Can you work these out from the model? Positions are in its coordinate system, mm. A direction names the side the tool comes from. Give positions to 0.01 mm unless a question says otherwise; leave off trailing zeros. Loops run counter-clockwise (first coordinate to the right, second up) from the corner with the lowest first, then second, coordinate; pieces in that order, holes last. Notation, with made-up numbers: (6, 63.25) - (16, 63.25) arc R24 cw to (16, 88.25) - close; hole circle Ø7 at (75.25, 50). An arc over 180 degrees is marked (long way). Answer as a JSON object with one key per item and string values.
```python
from build123d import *

# Parameters (mm, degrees)
F0_R     = 10.9982
F1_DEPTH = 7.0104
F2_R     = 1.27
F3_R     = 1.27


with BuildPart() as f1:
    # F0 (on Front) → F1 (new body)
    with BuildSketch(Plane.XZ):
        Polygon((-12.7, 9.9571658781), (-12.7, 5.2605122421), (-5.2605122421, 12.7), (-9.9571658781, 12.7), (-11.4818856978, 16.9197350247), (-28.3834853749, 28.3834853749), (-16.9197350247, 11.4818856978), align=None)
        Polygon((-16.0210356348, -1.9394766073), (-12.7, -5.2605122421), (-12.7, 5.2605122421), (-16.0210356348, 1.9394766073), (-20.0829786096, 3.8451401341), (-40.1403099645, 0), (-20.0829786096, -3.8451401341), align=None)
        Polygon((-9.9571658781, -12.7), (-5.2605122421, -12.7), (-12.7, -5.2605122421), (-12.7, -9.9571658781), (-16.9197350247, -11.4818856978), (-28.3834853749, -28.3834853749), (-11.4818856978, -16.9197350247), align=None)
        Polygon((1.9394766073, -16.0210356348), (5.2605122421, -12.7), (-5.2605122421, -12.7), (-1.9394766073, -16.0210356348), (-3.8451401341, -20.0829786096), (0, -40.1403099645), (3.8451401341, -20.0829786096), align=None)
        Polygon((12.7, -5.2605122421), (5.2605122421, -12.7), (9.9571658781, -12.7), (11.4818856978, -16.9197350247), (28.3834853749, -28.3834853749), (16.9197350247, -11.4818856978), (12.7, -9.9571658781), align=None)
        Polygon((12.7, 5.2605122421), (12.7, -5.2605122421), (16.0210356348, -1.9394766073), (20.0829786096, -3.8451401341), (40.1403099645, 0), (20.0829786096, 3.8451401341), (16.0210356348, 1.9394766073), align=None)
        Polygon((5.2605122421, 12.7), (12.7, 5.2605122421), (12.7, 9.9571658781), (16.9197350247, 11.4818856978), (28.3834853749, 28.3834853749), (11.4818856978, 16.9197350247), (9.9571658781, 12.7), align=None)
        Polygon((-5.2605122421, 12.7), (5.2605122421, 12.7), (1.9394766073, 16.0210356348), (3.8451401341, 20.0829786096), (0, 40.1403099645), (-3.8451401341, 20.0829786096), (-1.9394766073, 16.0210356348), align=None)
        Polygon((-5.2605122421, -12.7), (5.2605122421, -12.7), (12.7, -5.2605122421), (12.7, 5.2605122421), (5.2605122421, 12.7), (-5.2605122421, 12.7), (-12.7, 5.2605122421), (-12.7, -5.2605122421), align=None)
        Circle(F0_R, mode=Mode.SUBTRACT)
    extrude(amount=F1_DEPTH)

    # F2
    f2_edges = [f1.edges().sort_by_distance(p)[0] for p in [
        (-1.92257, -7.0104, -30.111644),
        (1.92257, -7.0104, -30.111644),
        (2.892308, -7.0104, -18.052007),
        (3.599994, -7.0104, -14.360518),
        (7.608839, -7.0104, -12.7),
        (10.719526, -7.0104, -14.809868),
        (19.932686, -7.0104, -22.65161),
        (22.65161, -7.0104, -19.932686),
        (14.809868, -7.0104, -10.719526),
        (12.7, -7.0104, -7.608839),
        (14.360518, -7.0104, -3.599994),
        (18.052007, -7.0104, -2.892308),
        (30.111644, -7.0104, -1.92257),
        (30.111644, -7.0104, 1.92257),
        (18.052007, -7.0104, 2.892308),
        (14.360518, -7.0104, 3.599994),
        (12.7, -7.0104, 7.608839),
        (14.809868, -7.0104, 10.719526),
        (22.65161, -7.0104, 19.932686),
        (19.932686, -7.0104, 22.65161),
        (10.719526, -7.0104, 14.809868),
        (7.608839, -7.0104, 12.7),
        (3.599994, -7.0104, 14.360518),
        (2.892308, -7.0104, 18.052007),
        (1.92257, -7.0104, 30.111644),
        (-1.92257, -7.0104, 30.111644),
        (-2.892308, -7.0104, 18.052007),
        (-3.599994, -7.0104, 14.360518),
        (-7.608839, -7.0104, 12.7),
        (-10.719526, -7.0104, 14.809868),
        (-19.932686, -7.0104, 22.65161),
        (-22.65161, -7.0104, 19.932686),
        (-14.809868, -7.0104, 10.719526),
        (-12.7, -7.0104, 7.608839),
        (-14.360518, -7.0104, 3.599994),
        (-18.052007, -7.0104, 2.892308),
        (-30.111644, -7.0104, 1.92257),
        (-19.932686, -7.0104, -22.65161),
        (-10.719526, -7.0104, -14.809868),
        (-7.608839, -7.0104, -12.7),
        (-3.599994, -7.0104, -14.360518),
        (-22.65161, -7.0104, -19.932686),
        (-14.809868, -7.0104, -10.719526),
        (-12.7, -7.0104, -7.608839),
        (-14.360518, -7.0104, -3.599994),
        (-18.052007, -7.0104, -2.892308),
        (-30.111644, -7.0104, -1.92257),
        (-2.892308, -7.0104, -18.052007),
    ]]
    fillet(f2_edges, radius=F2_R)

    # F3
    f3_edges = [f1.edges().sort_by_distance(p)[0] for p in [
        (19.932686, 0, 22.65161),
        (22.65161, 0, 19.932686),
        (14.809868, 0, 10.719526),
        (10.719526, 0, 14.809868),
        (7.608839, 0, 12.7),
        (3.599994, 0, 14.360518),
        (2.892308, 0, 18.052007),
        (1.92257, 0, 30.111644),
        (-1.92257, 0, 30.111644),
        (-2.892308, 0, 18.052007),
        (-3.599994, 0, 14.360518),
        (-7.608839, 0, 12.7),
        (-10.719526, 0, 14.809868),
        (-19.932686, 0, 22.65161),
        (-22.65161, 0, 19.932686),
        (-14.809868, 0, 10.719526),
        (-12.7, 0, 7.608839),
        (-14.360518, 0, 3.599994),
        (-18.052007, 0, 2.892308),
        (-30.111644, -5.7404, 1.92257),
        (-30.111644, 0, -1.92257),
        (-18.052007, 0, -2.892308),
        (-14.360518, 0, -3.599994),
        (-12.7, 0, -7.608839),
        (-14.809868, 0, -10.719526),
        (-22.65161, -5.7404, -19.932686),
        (-19.932686, 0, -22.65161),
        (-10.719526, 0, -14.809868),
        (-7.608839, 0, -12.7),
        (-3.599994, 0, -14.360518),
        (-2.892308, -5.7404, -18.052007),
        (-1.92257, 0, -30.111644),
        (1.92257, 0, -30.111644),
        (2.892308, 0, -18.052007),
        (3.599994, 0, -14.360518),
        (7.608839, 0, -12.7),
        (10.719526, 0, -14.809868),
        (19.932686, 0, -22.65161),
        (22.65161, 0, -19.932686),
        (14.809868, 0, -10.719526),
        (12.7, 0, -7.608839),
        (14.360518, 0, -3.599994),
        (18.052007, 0, -2.892308),
        (30.111644, 0, -1.92257),
        (30.111644, 0, 1.92257),
        (18.052007, 0, 2.892308),
        (14.360518, 0, 3.599994),
        (12.7, 0, 7.608839),
    ]]
    fillet(f3_edges, radius=F3_R)


solid = f1.part
```
1) I'm going to push flat-ended pins straight in: P1, Ø3, axis at x = -5.5, y = -4.5, coming from the +Z side; P2, Ø2, axis at y = -2.5, z = 8, coming from the +X side; P3, Ø3.5, axis at x = 8, y = -3, coming from the +Z side. Where does each tip first touch, or does it pass through?
Check sheet entries:
{"P1": "z = 13.96", "P2": "x = 12.7", "P3": "z = 12.7"}
2) If we mould it in two halves opening along Z, with no side actions, what happens to faces 5 (the flat face through (-10, 0, -7)), 6 (the cylindrical face through (-1.68, -0.36, -29.33)), 7 (the flat face through (3.58, -3.47, -14.38))? For each: released by +Z, released by -Z, zero draft, split by the parting line, or undercut.
Check sheet entries:
{"face 5": "zero draft", "face 6": "released by -Z", "face 7": "undercut"}
3) Which directions (+Z, -Z, +X, -X, +Y, -Y) give clear straight access to the entire face, cutting with the end or side of a thin tool? Please do faces 1 (the cylindrical face through (-10.9, -0.4, 14.3)), 2 (the flat face through (8, -3, -12.7)), 3 (the cylindrical face through (-10.914, -0.362, -14.225)), 4 (the cylindrical face through (-3.245, -6.628, 14.203)).
Check sheet entries:
{"face 1": "+Z, +Y", "face 2": "-Z, +Y, -Y", "face 3": "-Z, +Y", "face 4": "-Y"}
4) Imagine slicing it at A-A on x = -7.5. Write out the boundary of the cut face in (y, z), and give its area (3 significant figures).
Check sheet entries:
{"outline": "(-7.01, -11.43) arc R1.27 ccw to (-5.74, -12.7) - (-1.27, -12.7) arc R1.27 ccw to (0, -11.43) - (0, -8.04) - (-7.01, -8.04) - close; (-7.01, 8.04) - (0, 8.04) - (0, 11.43) arc R1.27 ccw to (-1.27, 12.7) - (-5.74, 12.7) arc R1.27 ccw to (-7.01, 11.43) - close", "area": "63.9 mm2"}
5) I need wall thicknesses on L1, parallel to X at y = -0.75, z = -21.5; L2, parallel to Z at x = 17, y = -3.75; L3, parallel to Z at x = 18.5, y = -6.25. Which ranges of each line are inside material? Lowest first, please.
Check sheet entries:
{"L1": "-23.71 to -18.43, -3.46 to 3.46, 18.43 to 23.58", "L2": "-20.66 to -11.6, -2.4 to 2.4, 11.6 to 20.66", "L3": "-21.55 to -14, -2.98 to 2.98, 14 to 21.55"}
6) Imagine slicing it at B-B on x = 18. Give the number of separate pieces and of enclosed holes in the cut face, and give its area (3 significant figures).
Check sheet entries:
{"separate pieces": "3", "enclosed holes": "0", "area": "150 mm2"}
